Input: dimensioned drawing with shaded views. Units: mm. Origin: part minimum x, y, z. Give positions to 0.01 mm unless a question says otherwise; leave off trailing zeros. Write each loop counter-clockwise with the first axis right and the second up, starting at its lowest first coordinate (ties: lowest second). Pieces come first, ordered by that corner, then holes. Notation, with made-up numbers: (62.5, -5.75) -> (82.5, -5.75) arc R20 cw to (82.5, 7.25) -> close; hole circle Ø8 at (3, -26.75). An arc over 180 degrees is marked (long way). Answer as a JSON object with one key per item and string values. Group by question number.
(1) Material intervals for probe 1 along X at (y, z) = (77.5, 2.95) (1 decimal); probe 2 along Y at (x, z) = (63.5, 4.35) (1 decimal); probe 3 along Y at (x, z) = (45.5, 2.7), sorted ascending.
(2) Section query C-C on x = 33.5. Output: boundary loops of the cut face in (y, z).
(3) Contact query for a flat-ended pin moving along its axis: pin 1 Ø3 at (y, z) = (62.5, 2) entering from -X (1 decimal). Output: stop coordinate, or through.
(4) Section query B-B on y = 66.5. Output: boundary loops of the cut face in (x, z), plus the area to 3 significant figures.
(5) Section query A-A on z = 3.95. Output: boundary loops of the cut face in (x, y) (1 decimal), plus the area to 3 significant figures.
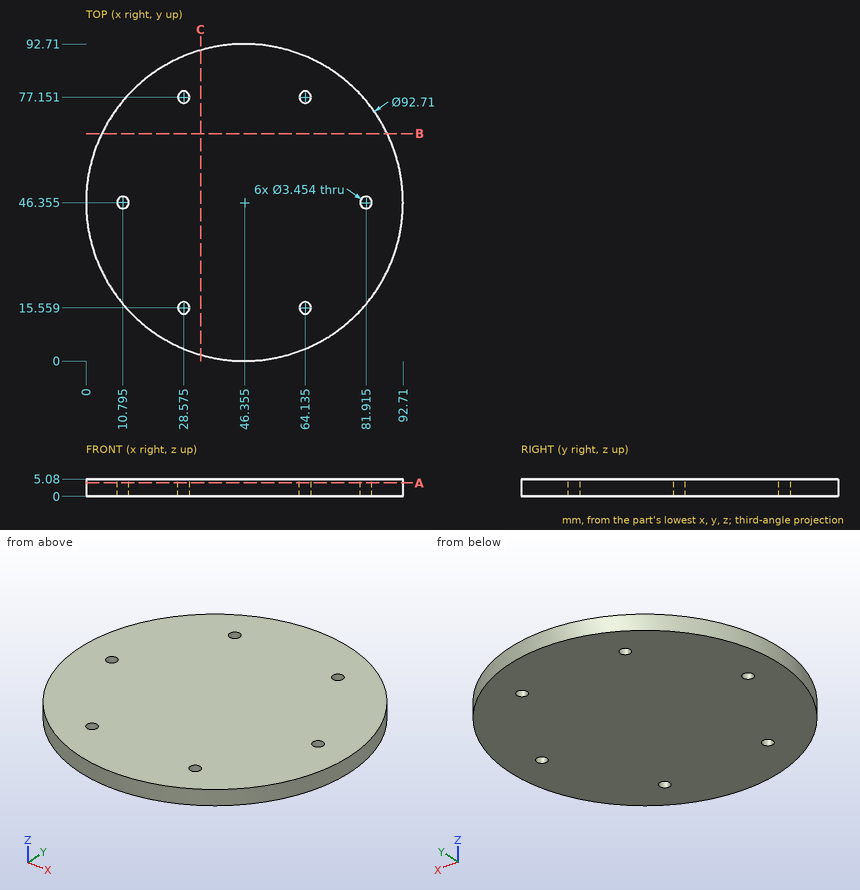
Answer list:
{
 "1": {"probe 1": "12 to 26.9, 30.3 to 62.4, 65.8 to 80.7", "probe 2": "3.3 to 14, 17.2 to 75.5, 78.8 to 89.4", "probe 3": "0.01 to 92.7"},
 "2": {"outline": "(1.82, 0) -> (90.89, 0) -> (90.89, 5.08) -> (1.82, 5.08) -> close"},
 "3": {"pin 1": "x = 2.4"},
 "4": {"outline": "(4.61, 0) -> (88.1, 0) -> (88.1, 5.08) -> (4.61, 5.08) -> close", "area": "424 mm2"},
 "5": {"outline": "circle Ø92.7 at (46.4, 46.4); hole circle Ø3.5 at (10.8, 46.4); hole circle Ø3.5 at (28.6, 15.6); hole circle Ø3.5 at (28.6, 77.2); hole circle Ø3.5 at (64.1, 15.6); hole circle Ø3.5 at (64.1, 77.2); hole circle Ø3.5 at (81.9, 46.4)", "area": "6,690 mm2"}
}
